Can you work these out from the drawing? Everything is in mm from the part's minimum corner. A direction names the side the tool comes from. Coordinates: 2 decimals unless noted, no trailing zeros. Loops run counter-clockwise (first coordinate to the right, second up) from the corner with the lowest first, then second, coordinate; pieces in that order, holes last. Notation, with made-up numbers: (-32.5, 83.5) - (19.5, 83.5) arc R23 cw to (19.5, 104.5) - close; hole circle Ø2 at (71.5, 46.25). An arc over 180 degrees is marked (long way). One line per question, with ' | ' between items. Start each with the question number.
1. We'd pull the mould along Y, two halves only. Please class the marked faces 4, 5, 6 and 7: pulls with the +Y half, pulls with the -Y half, needs draft (parallel to the pull), parting line crosses it, or undercut.
2. I want a section at D-D, the plane z = 49.5. Write out the boundary of the cut face in (x, y), then the cut area to 3 significant figures.
3. I want a section at B-B, the plane y = 46.5. Write out the boundary of the cut face in (x, z).
4. I'm going to push flat-ended pins straight in: P1, Ø5, axis at x = 18, y = 70.5, coming from the -Z side; P2, Ø4, axis at y = 26, z = 45.5, coming from the +X side; P3, Ø1.5, axis at x = 79, y = 29, coming from the -Z side. Where does each tip first touch, or does it pass through?
5. Which directions (+Z, -Z, +X, -X, +Y, -Y) give clear straight access to the entire face, cutting with the end or side of a thin tool? Please do the marked faces 1, 2 and 3.
6. I want a section at C-C, the plane x = 91. Write out the boundary of the cut face in (y, z).
7. Please list where these lines run through material, in increasing order: L1, parallel to X at y = 54, z = 34; L2, parallel to X at y = 18, z = 47.5; L3, parallel to Y at x = 9, z = 14. Write a range as [from, to].
8. I want a section at A-A, the plane z = 9.5. Write out the boundary of the cut face in (x, y), then the cut area to 3 significant figures.
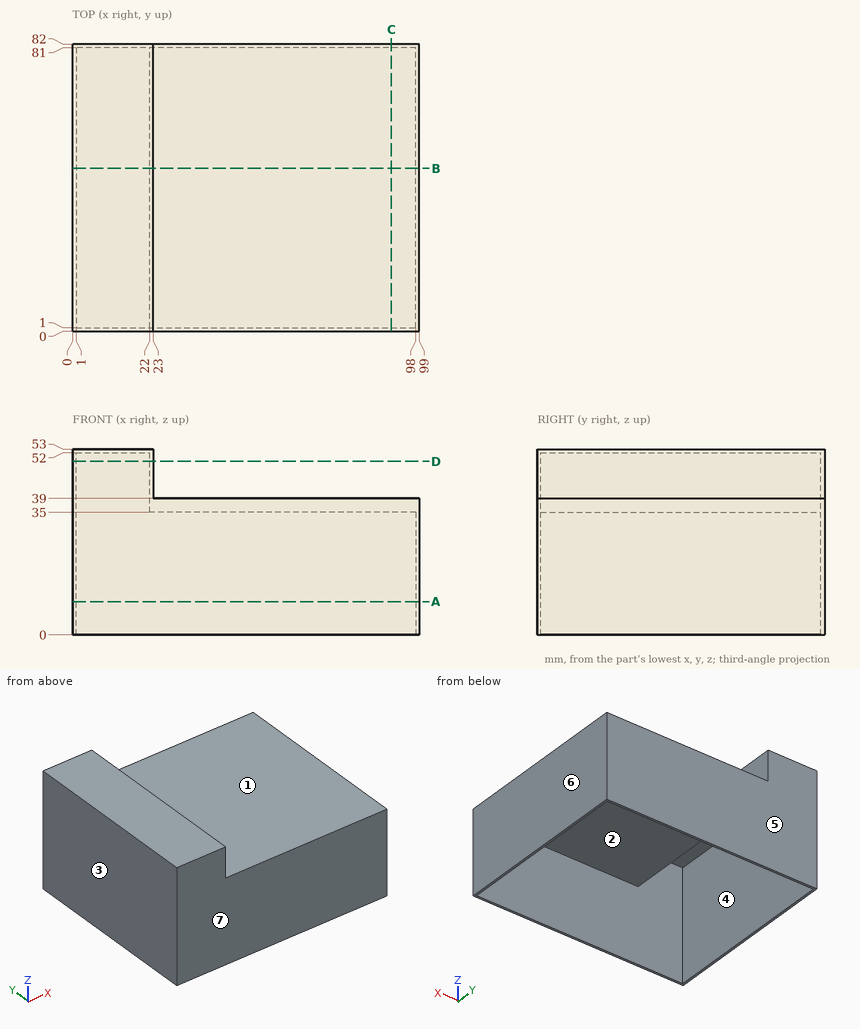
Results are:
1) face 4: undercut | face 5: pulls with the +Y half | face 6: needs draft | face 7: pulls with the -Y half
2) outline: (0, 0) - (23, 0) - (23, 82) - (0, 82) - close; hole (1, 1) - (22, 1) - (22, 81) - (1, 81) - close | area: 206 mm2
3) outline: (0, 0) - (1, 0) - (1, 52) - (22, 52) - (22, 35) - (98, 35) - (98, 0) - (99, 0) - (99, 39) - (23, 39) - (23, 53) - (0, 53) - close
4) P1: stops at z = 52 | P2: stops at x = 23 | P3: stops at z = 35
5) face 1: +Z, +X, +Y, -Y | face 2: -Z | face 3: +Z, -Z, -X, +Y, -Y
6) outline: (0, 0) - (1, 0) - (1, 35) - (81, 35) - (81, 0) - (82, 0) - (82, 39) - (0, 39) - close
7) L1: x = [0, 1], [98, 99] | L2: x = [0, 1], [22, 23] | L3: y = [0, 1], [81, 82]
8) outline: (0, 0) - (99, 0) - (99, 82) - (0, 82) - close; hole (1, 1) - (98, 1) - (98, 81) - (1, 81) - close | area: 358 mm2
